Source: CAD feature listing. Evaluate the final solid. Frame: model axes, mm. Give positions to 0.01 mm unless a question says otherwise; leave off trailing zeros. Write each loop counter-clockwise with the first axis right and the second up, starting at its lowest first coordinate (ties: lowest second). Pieces come first, ordered by that corner, then holes. Notation, with made-up numbers: M -7.5,-13.75 L 37.5,-13.75 A21 cw 37.5,25.25 Z; hole C -23.5,58.25 d4. An arc over 180 degrees is marked long. Return JSON: item names as keys, results as strings.
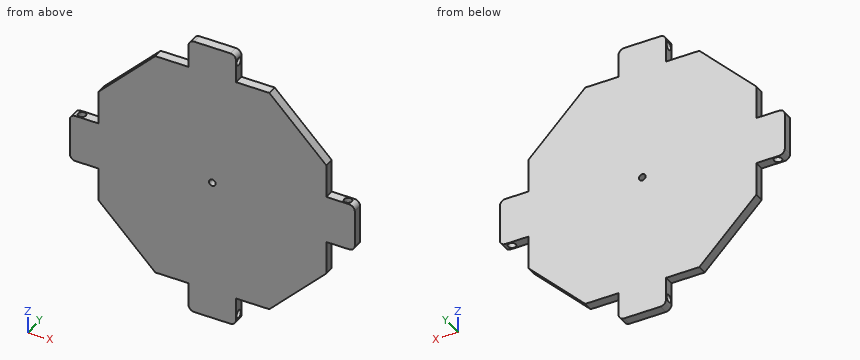
```python
from build123d import *

# Parameters (mm, degrees)
EXTRUDE_1_DEPTH     = 5
FILLET_1_R          = 3
SKETCH_7_R          = 1.75
CUT_EXTRUDE_5_DEPTH = 6
SKETCH_11_R         = 2
CUT_EXTRUDE_6_DEPTH = 88.5
SKETCH_12_R         = 2
CUT_EXTRUDE_7_DEPTH = 88.5


with BuildPart() as part:
    # 스케치1 → 보스-돌출1 (new body)
    with BuildSketch(Plane(origin=(0, 0, 0), x_dir=(1, 0, 0), z_dir=(0, 1, 0))):
        Polygon((-60, -30), (-30, -60), (-12.5, -60), (-12.5, -75), (12.5, -75), (12.5, -60), (30, -60), (60, -30), (60, -12.5), (75, -12.5), (75, 12.5), (60, 12.5), (60, 30), (30, 60), (12.5, 60), (12.5, 75), (-12.5, 75), (-12.5, 60), (-30, 60), (-60, 30), (-60, 12.5), (-75, 12.5), (-75, -12.5), (-60, -12.5), align=None)
    extrude(amount=EXTRUDE_1_DEPTH)

    # 필렛1
    fillet_1_edges = [part.edges().sort_by_distance(p)[0] for p in [
        (-12.5, 2.5, -75),
        (12.5, 2.5, -75),
        (75, 2.5, -12.5),
        (75, 2.5, 12.5),
        (12.5, 2.5, 75),
        (-12.5, 2.5, 75),
        (-75, 2.5, 12.5),
        (-75, 2.5, -12.5),
    ]]
    fillet(fillet_1_edges, radius=FILLET_1_R)

    # 스케치7 → 컷-돌출5 (cut, through all)
    with BuildSketch(Plane(origin=(0, 5, 0), x_dir=(1, 0, 0), z_dir=(0, 1, 0))):
        Circle(SKETCH_7_R)
    extrude(amount=-CUT_EXTRUDE_5_DEPTH, mode=Mode.SUBTRACT)

    # 스케치11 → 컷-돌출6 (cut, through all)
    with BuildSketch(Plane.XY.offset(12.5)):
        with Locations((-70, 2.5)):
            Circle(SKETCH_11_R)
        with Locations((70, 2.5)):
            Circle(SKETCH_11_R)
    extrude(amount=-CUT_EXTRUDE_6_DEPTH, mode=Mode.SUBTRACT)

    # 스케치12 → 컷-돌출7 (cut, through all)
    with BuildSketch(Plane.ZY.offset(12.5)):
        with Locations((-70, 2.5)):
            Circle(SKETCH_12_R)
        with Locations((70, 2.5)):
            Circle(SKETCH_12_R)
    extrude(amount=-CUT_EXTRUDE_7_DEPTH, mode=Mode.SUBTRACT)


solid = part.part
```
1) Cut plane B-B, the plane x = 0. Return the cut outline in (y, z).
Numbers:
{"outline": "M 0,-75 L 5,-75 L 5,-1.75 L 0,-1.75 Z; M 0,1.75 L 5,1.75 L 5,75 L 0,75 Z; hole C 2.5,-70 d4; hole C 2.5,70 d4"}
2) Cut plane A-A, the plane x = -70. Return the cut outline in (y, z).
Numbers:
{"outline": "M 0,-12.5 L 0.5,-12.5 L 0.5,12.5 L 0,12.5 Z; M 4.5,-12.5 L 5,-12.5 L 5,12.5 L 4.5,12.5 Z"}
3) Contact query for flat-ended pins moving along their axis: pin 1 Ø1.5 at (y, z) = (3.5, 66.5) entering from -X; pin 2 Ø1.5 at (y, z) = (3.5, 21) entering from +X; pin 3 Ø1.5 at (y, z) = (2, -64) entering from +X; pin 4 Ø3 at (y, z) = (2.5, 70) entering from -X. Output: stop coordinate, or through.
Numbers:
{"pin 1": "stops at x = -12.5", "pin 2": "stops at x = 60", "pin 3": "stops at x = 12.5", "pin 4": "passes through"}
4) Line query: line 1 (X direction, y = 2.1, z = 0); line 2 (X direction, y = 2.55, z = -7); line 3 (Z direction, x = 8.5, y = 3.1). Output: solid intervals per line, ascending. Write a range as [from, to].
Numbers:
{"line 1": "x = [-75, -71.96], [-68.04, -1.75], [1.75, 68.04], [71.96, 75]", "line 2": "x = [-75, -72], [-68, 68], [72, 75]", "line 3": "z = [-75, -71.91], [-68.09, 68.09], [71.91, 75]"}
5) Cut plane D-D, the plane y = 3.45. Give the number of separate pieces and of enclosed holes in the cut face, then the cut area to 3 significant figures.
Numbers:
{"separate pieces": "5", "enclosed holes": "1", "area": "13,700 mm²"}
6) Cut plane C-C, the plane z = -70. Return the cut outline in (x, y), then the cut area to 3 significant figures.
Numbers:
{"outline": "M -12.5,0 L 12.5,0 L 12.5,0.5 L -12.5,0.5 Z; M -12.5,4.5 L 12.5,4.5 L 12.5,5 L -12.5,5 Z", "area": "25.0 mm²"}
